Can you work these out from the drawing? Everything is in mm from the part's minimum corner. A direction names the side the tool comes from. Coordinates: 2 decimals unless noted, no trailing zeros. Loops run counter-clockwise (first coordinate to the right, second up) from the corner with the lowest first, then second, coordinate; pieces in that order, holes last.
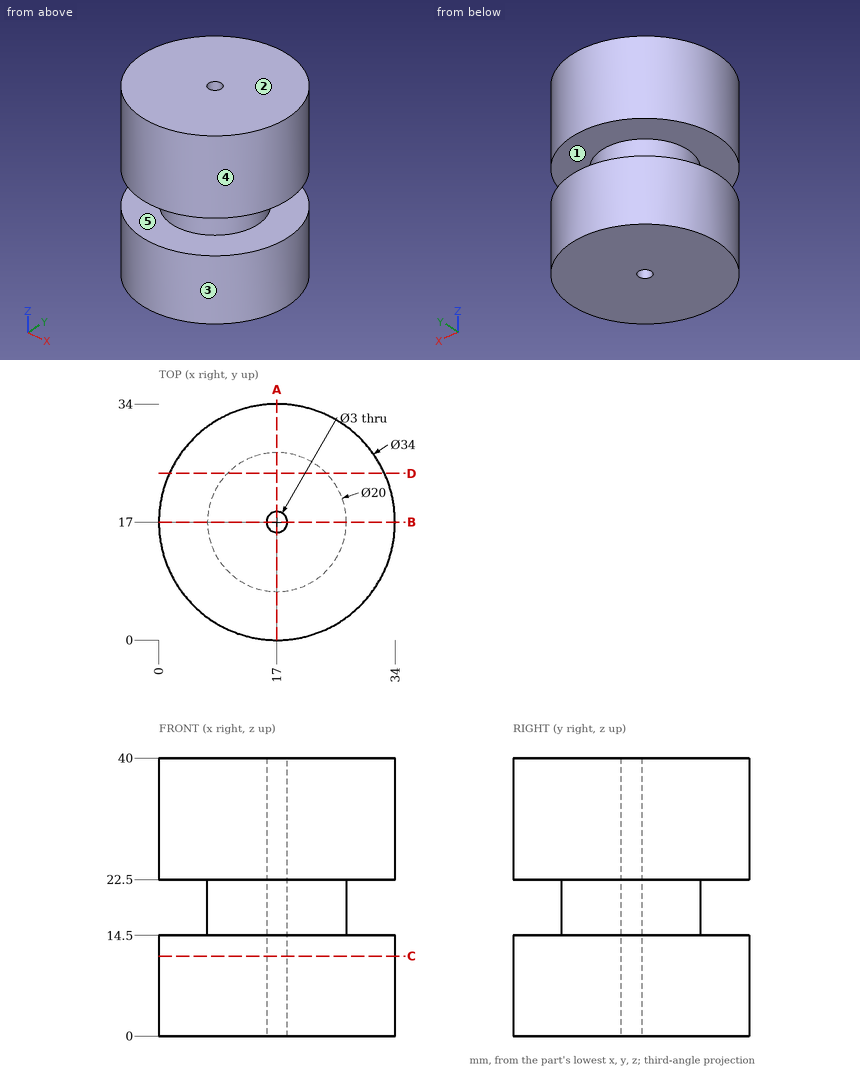
(1) We'd pull the mould along Z, two halves only. Please class the marked faces 1, 2 and 3: +Z half, -Z half, draft (parallel to the pull), parting line (faces both ways), or undercut.
Answers:
face 1: undercut
face 2: +Z half
face 3: draft
(2) For pin 1 (12 mm diameter, centred on y = 29.5, z = 33.5, fed in from +X); pin 2 (1 mm diameter, centred on y = 8.5, z = 23, fed in from +X); pin 3 (3 mm diameter, centred on y = 9, z = 29, fed in from -X), each with a flat end and sliding along its axis, tell me the tip position at first contact or that it passes through.
Answers:
pin 1: stops at x = 32.71
pin 2: stops at x = 32
pin 3: stops at x = 1.29
(3) Which directions (+Z, -Z, +X, -X, +Y, -Y) give clear straight access to the entire face, cutting with the end or side of a thin tool? Please do the marked faces 4 and 5.
Answers:
face 4: +Z, -Z
face 5: none
(4) I need wall thicknesses on probe 1 along Z at (x, y) = (2.5, 25); probe 2 along Y at (x, z) = (17, 18); probe 3 along Y at (x, z) = (17, 30). Which ranges of each line are inside material? Lowest first, please.
Answers:
probe 1: z = 0 to 14.5, 22.5 to 40
probe 2: y = 7 to 15.5, 18.5 to 27
probe 3: y = 0 to 15.5, 18.5 to 34
(5) Imagine slicing it at D-D, the plane y = 24. Write out the boundary of the cut face in (x, z), and give its area (3 significant figures).
Answers:
outline: (1.51, 0) - (32.49, 0) - (32.49, 14.5) - (24.14, 14.5) - (24.14, 22.5) - (32.49, 22.5) - (32.49, 40) - (1.51, 40) - (1.51, 22.5) - (9.86, 22.5) - (9.86, 14.5) - (1.51, 14.5) - close
area: 1,110 mm2
(6) Imagine slicing it at C-C, the plane z = 11.5. Write out the boundary of the cut face in (x, y), and give its area (3 significant figures).
Answers:
outline: circle Ø34 at (17, 17); hole circle Ø3 at (17, 17)
area: 901 mm2
(7) Imagine slicing it at A-A, the plane x = 17. Write out the boundary of the cut face in (y, z).
Answers:
outline: (0, 0) - (15.5, 0) - (15.5, 40) - (0, 40) - (0, 22.5) - (7, 22.5) - (7, 14.5) - (0, 14.5) - close; (18.5, 0) - (34, 0) - (34, 14.5) - (27, 14.5) - (27, 22.5) - (34, 22.5) - (34, 40) - (18.5, 40) - close
